Input: part model. Units: mm. Frame: model coordinates. A direction names the side the tool comes from. Give positions to 0.01 mm unless a question says otherwise; leave off trailing zeros. Write each loop counter-clockwise with the first axis right and the second up, starting at its lowest first coordinate (ties: lowest second). Pieces come first, ordered by that corner, then holes. Notation, with made-up numbers: (79.25, 15.5) -> (111.25, 15.5) arc R6 ccw to (111.25, 20.5) -> close; hole circle Ø6 at (-31.75, 41). An arc over 180 degrees is marked (long way). Answer as a JSON object with one key per item and string values. Group by question number.
from build123d import *

# Parameters (mm, degrees)
SKETCH1_W                      = 60
SKETCH1_H                      = 57
BOSS_EXTRUDE1_DEPTH            = 3
F_4_5_4_5_DIAMETER_HOLE1_D     = 4.5
F_4_5_4_5_DIAMETER_HOLE1_DEPTH = 15
F_4_5_4_5_DIAMETER_HOLE1_TIP   = 1.351936393
SKETCH4_W                      = 20
SKETCH4_H                      = 20
BOSS_EXTRUDE2_DEPTH            = 3
F_2_7_2_7_DIAMETER_HOLE1_D     = 2.7
F_2_7_2_7_DIAMETER_HOLE1_DEPTH = 15
F_2_7_2_7_DIAMETER_HOLE1_TIP   = 0.811161836
FILLET1_R                      = 2


with BuildPart() as part:
    # Sketch1 → Boss-Extrude1 (new body)
    with BuildSketch(Plane(origin=(0, 0, 0), x_dir=(1, 0, 0), z_dir=(0, 1, 0))):
        Rectangle(SKETCH1_W, SKETCH1_H)
    extrude(amount=BOSS_EXTRUDE1_DEPTH)

    # Ø4.5 (4.5) Diameter Hole1
    with Locations(Plane(origin=(0, 3, 0), x_dir=(1, 0, 0), z_dir=(0, 1, 0))):
        with Locations((-25.437, 0), (-6.687, 0), (12.063, 18.75), (12.063, -18.75)):
            Hole(F_4_5_4_5_DIAMETER_HOLE1_D / 2, depth=F_4_5_4_5_DIAMETER_HOLE1_DEPTH)
            with Locations((0, 0, -(F_4_5_4_5_DIAMETER_HOLE1_DEPTH + F_4_5_4_5_DIAMETER_HOLE1_TIP / 2))):  # 118° drill point
                Cone(0, F_4_5_4_5_DIAMETER_HOLE1_D / 2, F_4_5_4_5_DIAMETER_HOLE1_TIP, mode=Mode.SUBTRACT)

    # Sketch4 → Boss-Extrude2 (add)
    with BuildSketch(Plane(origin=(0, 3, 0), x_dir=(1, 0, 0), z_dir=(0, 1, 0))):
        with Locations((40, 8.5)):
            Rectangle(SKETCH4_W, SKETCH4_H)
    extrude(amount=-BOSS_EXTRUDE2_DEPTH)

    # Ø2.7 (2.7) Diameter Hole1
    with Locations(Plane(origin=(0, 3, 0), x_dir=(1, 0, 0), z_dir=(0, 1, 0))):
        with Locations((40, 13.5), (40, 3.5)):
            Hole(F_2_7_2_7_DIAMETER_HOLE1_D / 2, depth=F_2_7_2_7_DIAMETER_HOLE1_DEPTH)
            with Locations((0, 0, -(F_2_7_2_7_DIAMETER_HOLE1_DEPTH + F_2_7_2_7_DIAMETER_HOLE1_TIP / 2))):  # 118° drill point
                Cone(0, F_2_7_2_7_DIAMETER_HOLE1_D / 2, F_2_7_2_7_DIAMETER_HOLE1_TIP, mode=Mode.SUBTRACT)

    # Fillet1
    fillet1_edges = [part.edges().sort_by_distance(p)[0] for p in [
        (30, 1.5, 1.5),
        (30, 1.5, -18.5),
        (50, 1.5, -18.5),
        (50, 1.5, 1.5),
        (30, 1.5, 28.5),
        (-30, 1.5, 28.5),
        (-30, 1.5, -28.5),
        (30, 1.5, -28.5),
    ]]
    fillet(fillet1_edges, radius=FILLET1_R)


solid = part.part
1. Contact query for flat-ended pins moving along their axis: pin 1 Ø1.5 at (y, z) = (2, -23) entering from +X; pin 2 Ø4 at (x, z) = (-6.687, 0) entering from -Y; pin 3 Ø0.9 at (x, y) = (42.5, 2) entering from +Z. Output: stop coordinate, or through.
2. Section B-B (x = 40). Return the cut outline in (y, z), plus the area to 3 significant figures.
3. Mould query, pull axis X, two halves, no side actions, for faces 3 (the face through (41.35, 1.48, -3.56)), 4 (the face through (40, 2, 1.5)), 5 (the face through (-29.43, 1.52, 27.9)), 6 (the face through (30.57, 1.48, -19.1)). Classes: pulls with the +X half, pulls with the -X half, needs draft (parallel to the pull), parting line crosses it, or undercut.
4. Section C-C (y = 2). Return the cut outline in (x, z), plus the area to 3 significant figures.
5. Section D-D (x = -8). Return the cut outline in (y, z), plus the area to 3 significant figures.
6. Section A-A (z = 18.75). Return the cut outline in (x, y).
7. Reachability of faces 1 (the face through (40, 2, -18.5)), 2 (the face through (12.551, 1.479, 20.946)) from +Z, -Z, +X, -X, +Y, -Y: full face, straight path, thin tool, end or side. Return the list, or none.
8. Line query: line 1 (Z direction, x = 40, y = 1.7); line 2 (X direction, y = 0.7, z = -13.5); line 3 (Z direction, x = -25.5, y = 0.25). Output: solid intervals per line, ascending.
Working result:
{
 "1": {"pin 1": "stops at x = 30", "pin 2": "passes through", "pin 3": "stops at z = 1.5"},
 "2": {"outline": "(0, -18.5) -> (3, -18.5) -> (3, -14.85) -> (0, -14.85) -> close; (0, -12.15) -> (3, -12.15) -> (3, -4.85) -> (0, -4.85) -> close; (0, -2.15) -> (3, -2.15) -> (3, 1.5) -> (0, 1.5) -> close", "area": "43.8 mm^2"},
 "3": {"face 3": "undercut", "face 4": "needs draft", "face 5": "pulls with the -X half", "face 6": "pulls with the +X half"},
 "4": {"outline": "(-30, -26.5) arc R2 ccw to (-28, -28.5) -> (28, -28.5) arc R2 ccw to (30, -26.5) -> (30, -20.5) arc R2 cw to (32, -18.5) -> (48, -18.5) arc R2 ccw to (50, -16.5) -> (50, -0.5) arc R2 ccw to (48, 1.5) -> (32, 1.5) arc R2 cw to (30, 3.5) -> (30, 26.5) arc R2 ccw to (28, 28.5) -> (-28, 28.5) arc R2 ccw to (-30, 26.5) -> close; hole circle Ø4.5 at (-25.44, 0); hole circle Ø4.5 at (-6.69, 0); hole circle Ø4.5 at (12.06, -18.75); hole circle Ø4.5 at (12.06, 18.75); hole circle Ø2.7 at (40, -13.5); hole circle Ø2.7 at (40, -3.5)", "area": "3,740 mm^2"},
 "5": {"outline": "(0, -28.5) -> (3, -28.5) -> (3, -1.83) -> (0, -1.83) -> close; (0, 1.83) -> (3, 1.83) -> (3, 28.5) -> (0, 28.5) -> close", "area": "160 mm^2"},
 "6": {"outline": "(-30, 0) -> (9.81, 0) -> (9.81, 3) -> (-30, 3) -> close; (14.31, 0) -> (30, 0) -> (30, 3) -> (14.31, 3) -> close"},
 "7": {"face 1": "-Z, +X, +Y, -Y", "face 2": "+Y, -Y"},
 "8": {"line 1": "z = -18.5 to -14.85, -12.15 to -4.85, -2.15 to 1.5", "line 2": "x = -30 to 38.65, 41.35 to 50", "line 3": "z = -28.5 to -2.25, 2.25 to 28.5"}
}
